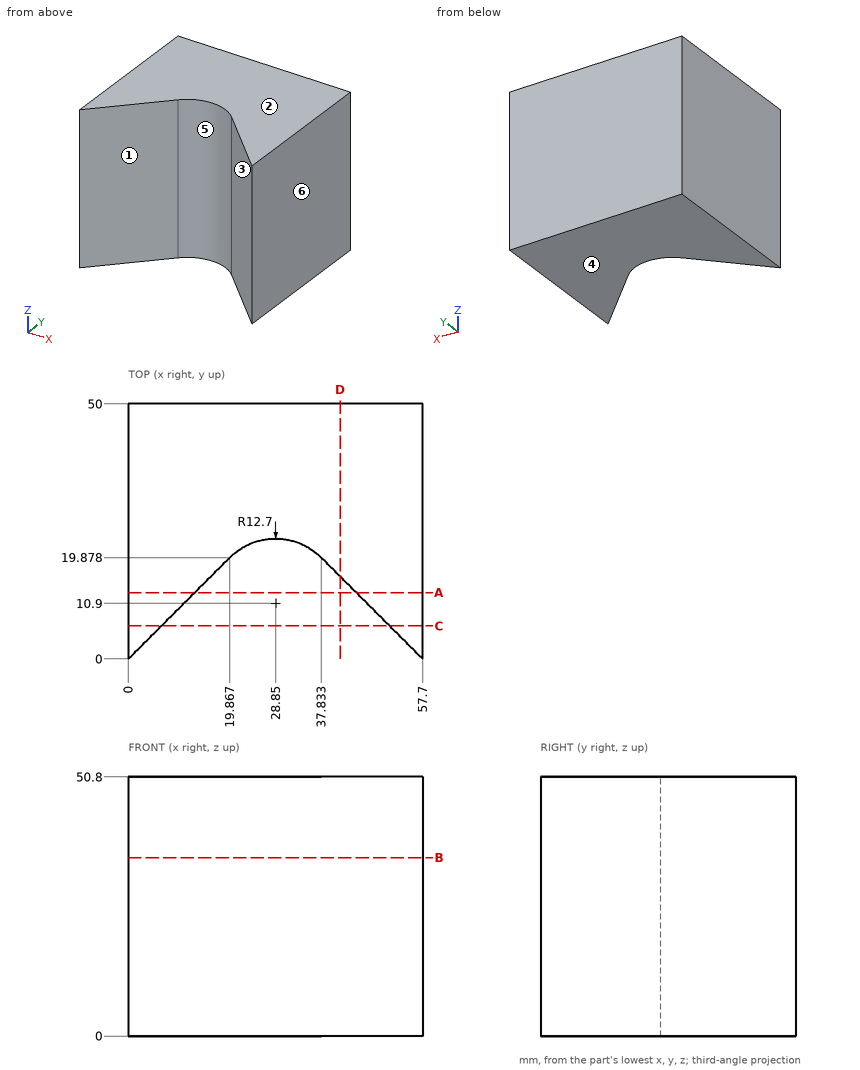
Check sheet for the drawn part. Datum: minimum x, y, z corner. Units: mm. A direction names the side the tool comes from. Coordinates: 2 decimals unless noted, no trailing zeros. Loops run counter-clockwise (first coordinate to the right, second up) from the corner with the lowest first, then second, coordinate; pieces in that order, holes last. Notation, with made-up numbers: (-3, -30.5) -> (26, -30.5) arc R26 ccw to (26, -3.5) -> close; hole circle Ø2 at (-38.5, -39). An arc over 180 degrees is marked (long way). Answer in a Markdown table with one row per item.
1. Access from +Z, -Z, +X, -X, +Y, -Y to the whole of each face (thin tool, end or side, straight path). Record for the marked faces 1 and 2.
Check values:
| item | result |
|---|---|
| face 1 | +Z, -Z, -Y |
| face 2 | +Z, +X, -X, +Y, -Y |
2. Go/stop test with flat-tipped pins: pin 1 (6 mm diameter, centred on y = 28.5, z = 44, fed in from -X); pin 2 (4 mm diameter, centred on x = 38.5, z = 16, fed in from -Y). Record where each tip stops, or that it passes through.
Check values:
| item | result |
|---|---|
| pin 1 | stops at x = 0 |
| pin 2 | stops at y = 17.21 |
3. Sectioned sample at C-C, the plane y = 6.5. Record the boundary of the cut face in (x, z), then the cut area to 3 significant figures.
Check values:
| item | result |
|---|---|
| outline | (0, 0) -> (6.5, 0) -> (6.5, 50.8) -> (0, 50.8) -> close; (51.2, 0) -> (57.7, 0) -> (57.7, 50.8) -> (51.2, 50.8) -> close |
| area | 660 mm2 |
4. Material ranges on line 1 along X through (y, z) = (16, 33); line 2 along X through (y, z) = (3.5, 11); line 3 along Y through (x, z) = (41, 4), recorded low to high. Write a range as [from, to].
Check values:
| item | result |
|---|---|
| line 1 | x = [0, 15.99], [41.71, 57.7] |
| line 2 | x = [0, 3.5], [54.2, 57.7] |
| line 3 | y = [16.71, 50] |
5. Sectioned sample at A-A, the plane y = 13. Record the boundary of the cut face in (x, z).
Check values:
| item | result |
|---|---|
| outline | (0, 0) -> (12.99, 0) -> (12.99, 50.8) -> (0, 50.8) -> close; (44.71, 0) -> (57.7, 0) -> (57.7, 50.8) -> (44.71, 50.8) -> close |
6. Sectioned sample at D-D, the plane x = 41.5. Record the boundary of the cut face in (y, z), then the cut area to 3 significant figures.
Check values:
| item | result |
|---|---|
| outline | (16.21, 0) -> (50, 0) -> (50, 50.8) -> (16.21, 50.8) -> close |
| area | 1,720 mm2 |
7. Release check for a two-part mould opening along X. For the marked faces 3, 4, 5 and 6 record: released by +X, released by -X, zero draft, split by the parting line, or undercut.
Check values:
| item | result |
|---|---|
| face 3 | undercut |
| face 4 | zero draft |
| face 5 | undercut |
| face 6 | released by +X |
8. Sectioned sample at B-B, the plane z = 35. Record the boundary of the cut face in (x, y).
Check values:
| item | result |
|---|---|
| outline | (0, 0) -> (19.87, 19.88) arc R12.7 cw to (37.83, 19.88) -> (57.7, 0) -> (57.7, 50) -> (0, 50) -> close |
